CAD build for the part. Positions are in the model's coordinates, mm. A direction names the side the tool comes from. Give positions to 0.01 mm unless a question says otherwise; leave off trailing zeros. Write each loop counter-clockwise with the first axis right and the second up, starting at its lowest first coordinate (ties: lowest second). Pieces come first, ordered by that corner, then holes. Notation, with made-up numbers: M -1.75,39 L 21.25,39 A7 cw 21.25,43 Z; hole C 22,42 d8. An arc over 180 degrees is marked long. One line per question, with ' | ' between items. Start each with the question number.
1. Which spindle directions (+Z, -Z, +X, -X, +Y, -Y) get a long thin tool onto all of the face, cutting with end or side? Do faces 4 (the face through (1, 35, 6)), 5 (the face through (23.846, -7.509, 4.93)). Say none if no direction does.
2. Flat gauge pin, fed straight in: pin 1 (6 mm diameter, centred on x = -27.5, y = 8, fed in from -Z). Where does the tip first touch, or does it go through?
3. Cut at D-D, the plane y = -16. Write the cut outline in (x, z).
4. Cut at C-C, the plane z = 4. Write the cut outline in (x, y).
5. Cut at A-A, the plane x = 0. Write the cut outline in (y, z), then the cut area to 3 significant figures.
6. Cut at B-B, the plane y = 0. Write the cut outline in (x, z), then the cut area to 4 significant figures.
7. Wall check: L1, parallel to Y at x = 1, z = 9.25; L2, parallel to Y at x = 0, z = 10.85; L3, parallel to Z at x = 23, y = -8. Give the ranges that are in metal, low to high.
8. Pull direction Y, two halves, no side cores. Call faces 1 (the face through (-1, -35, 6)), 2 (the face through (-0.54, 2.44, 11.48)), 3 (the face through (-75, 0, 6)): released by +Y, released by -Y, zero draft, split by the parting line, or undercut.
Autodesk Inventor part; units mm, degrees
ref_plane "YZ Plane" through (0, 0, 0) normal (1, 0, 0) x (0, 1, 0)
ref_plane "XZ Plane" through (0, 0, 0) normal (0, 1, 0) x (-1, 0, 0)
ref_plane "XY Plane" through (0, 0, 0) normal (0, 0, 1) x (1, 0, 0)
sketch "Sketch1" plane through (0, 0, 0) normal (0, 0, 1) x (1, 0, 0)
  circle A0 centre (0, 0) radius 25
  line L0 (-75, -35) -> (75, -35)
  line L1 (75, -35) -> (75, 35)
  line L2 (75, 35) -> (-75, 35)
  line L3 (-75, 35) -> (-75, -35)
  line L4 (-75, -35) -> (75, 35) construction
  line L5 (75, -35) -> (-75, 35) construction
  dimension "d0" = 50
  dimension "d2" = 70
  dimension "d3" = 150
extrude "Extrusion1" add sketch "Sketch1" along normal blind 10
sketch "Sketch3" plane through (75, -35, 0) normal (1, 0, 0) x (0, 0, -1)
  line L0 (-90, 0) -> (-90, 70)
  line L1 (-90, 35) -> (-50, 35) construction
  circle A0 centre (-50, 35) radius 25
  point P0 (0, 35)
  dimension "d10" = 50
  dimension "d11" = 40
extrude "Extrusion3" cut sketch "Sketch3" against normal through all
sketch "Sketch4" plane through (0, 0, 10) normal (0, 0, 1) x (1, 0, 0)
  line L0 (-75, 35) -> (-75, -35)
  line L1 (-75, -35) -> (75, -35)
  line L2 (75, -35) -> (75, 35)
  line L3 (75, 35) -> (-75, 35)
  circle A0 centre (0, 0) radius 25 construction
  circle A1 centre (0, 0) radius 2.5
  dimension "d14" = 5
extrude "Extrusion4" add sketch "Sketch4" along normal blind 3
properties part number "CamBracket"
Here are the results:
1) face 4: +Z, -Z, +X, -X, +Y | face 5: -Z
2) pin 1: z = 0
3) outline: M -75,0 L -19.21,0 L -19.21,10 L 19.21,10 L 19.21,0 L 75,0 L 75,13 L -75,13 Z
4) outline: M -75,-35 L 75,-35 L 75,35 L -75,35 Z; hole C 0,0 d50
5) outline: M -35,0 L -25,0 L -25,10 L -2.5,10 L -2.5,13 L -35,13 Z; M 2.5,10 L 25,10 L 25,0 L 35,0 L 35,13 L 2.5,13 Z | area: 395 mm^2
6) outline: M -75,0 L -25,0 L -25,10 L -2.5,10 L -2.5,13 L -75,13 Z; M 2.5,10 L 25,10 L 25,0 L 75,0 L 75,13 L 2.5,13 Z | area: 1,435 mm^2
7) L1: -35 to -24.98, 24.98 to 35 | L2: -35 to -2.5, 2.5 to 35 | L3: 10 to 13
8) face 1: released by -Y | face 2: undercut | face 3: zero draft
